from build123d import *

# Parameters (mm, degrees)
SKETCH1_R           = 2.75
BOSS_EXTRUDE1_DEPTH = 6.35
FILLET1_R           = 6.35
CHAMFER1_SIZE       = 3.175
SKETCH2_W           = 234.95
SKETCH2_H           = 12.7
BOSS_EXTRUDE2_DEPTH = 6.35


with BuildPart() as part:
    # Sketch1 → Boss-Extrude1 (new body)
    with BuildSketch(Plane.XY):
        with BuildLine():
            ThreePointArc((-19.05, 19.05), (-31.75, 6.35), (-19.05, -6.35))
            Line((-19.05, -6.35), (-19.05, -260.35))
            ThreePointArc((-19.05, -260.35), (-31.75, -273.05), (-19.05, -285.75))
            Line((-19.05, -285.75), (241.3, -285.75))
            ThreePointArc((241.3, -285.75), (254, -273.05), (241.3, -260.35))
            Line((241.3, -260.35), (241.3, -6.35))
            ThreePointArc((241.3, -6.35), (254, 6.35), (241.3, 19.05))
            Line((241.3, 19.05), (-19.05, 19.05))
        make_face()
        with Locations((241.3, 6.35)):
            Circle(SKETCH1_R, mode=Mode.SUBTRACT)
        with Locations((-19.05, -273.05)):
            Circle(SKETCH1_R, mode=Mode.SUBTRACT)
        with Locations((-9.525, -276.225)):
            Circle(SKETCH1_R, mode=Mode.SUBTRACT)
        with Locations((231.775, -276.225)):
            Circle(SKETCH1_R, mode=Mode.SUBTRACT)
        with Locations((241.3, -273.05)):
            Circle(SKETCH1_R, mode=Mode.SUBTRACT)
        with BuildLine():
            Line((-6.35, -247.65), (-6.35, -19.05))
            ThreePointArc((-6.35, -19.05), (6.35, -6.35), (-6.35, 6.35))
            Line((-6.35, 6.35), (228.6, 6.35))
            Line((228.6, 6.35), (228.6, -273.05))
            Line((228.6, -273.05), (-6.35, -273.05))
            ThreePointArc((-6.35, -273.05), (6.35, -260.35), (-6.35, -247.65))
        make_face(mode=Mode.SUBTRACT)
        with Locations((-6.35, -6.35)):
            Circle(SKETCH1_R, mode=Mode.SUBTRACT)
        with Locations((-6.35, -260.35)):
            Circle(SKETCH1_R, mode=Mode.SUBTRACT)
        with Locations((-19.05, 6.35)):
            Circle(SKETCH1_R, mode=Mode.SUBTRACT)
        with Locations((-9.525, 9.525)):
            Circle(SKETCH1_R, mode=Mode.SUBTRACT)
        with Locations((231.775, 9.525)):
            Circle(SKETCH1_R, mode=Mode.SUBTRACT)
    extrude(amount=BOSS_EXTRUDE1_DEPTH)

    # Fillet1
    fillet1_edges = [part.edges().sort_by_distance(p)[0] for p in [
        (228.6, -273.05, 3.175),
        (228.6, 6.35, 3.175),
        (-6.35, 6.35, 3.175),
    ]]
    fillet(fillet1_edges, radius=FILLET1_R)
    fillet1_2_edges = [part.edges().sort_by_distance(p)[0] for p in [
        (-6.35, -273.05, 3.175),
    ]]
    fillet(fillet1_2_edges, radius=FILLET1_R)

    # Chamfer1
    chamfer1_edges = [part.edges().sort_by_distance(p)[0] for p in [
        (-21.8, 6.35, 0),
        (-21.8, -273.05, 0),
        (238.55, 6.35, 0),
        (238.55, -273.05, 0),
        (-9.1, -260.35, 0),
        (-9.1, -6.35, 0),
    ]]
    chamfer(chamfer1_edges, length=CHAMFER1_SIZE)

    # Sketch2 → Boss-Extrude2 (add)
    with BuildSketch(Plane.XY.offset(6.35)):
        with Locations((111.125, -133.35)):
            Rectangle(SKETCH2_W, SKETCH2_H)
    extrude(amount=-BOSS_EXTRUDE2_DEPTH)


solid = part.part
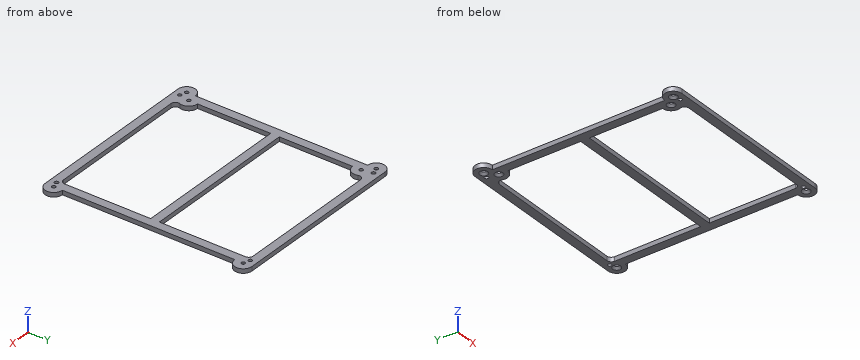
The listing builds one solid part. Answer for the finished solid, in the listing's coordinates (mm). Give positions to 0.01 mm unless a question says otherwise; leave off trailing zeros. Write each loop counter-clockwise with the first axis right and the second up, starting at its lowest first coordinate (ties: lowest second). Pieces come first, ordered by that corner, then holes. Notation, with made-up numbers: (52.25, 85) -> (90.25, 85) arc R20 cw to (90.25, 109) -> close; hole circle Ø10 at (6.5, 70.5). An arc over 180 degrees is marked (long way). One line per question, with ' | ' between items. Start each with the question number.
1. Find the intervals of material crossed by probe 1 along Y at (x, z) = (24, 0.75); probe 2 along X at (y, z) = (-126, 2.75), in increasing order.
2. Given pin 1 Ø7 at (x, y) = (241.3, 6.35) entering from -Z (3 decimals); pin 2 Ø3 at (y, z) = (-215.5, 4.5) entering from +X, each flat-ended and moving along its own axis, determine where each tip first touches the part or whether it passes through.
3. Section A-A (x = 210) is taken. Determine the outline of the cut face in (y, z).
4. Section B-B (y = -60.5) is taken. Determine the outline of the cut face in (x, z).
5. Section C-C (z = 4.75) is taken. State how many separate pieces and enclosed holes the cut face has, plus the area to 3 significant figures.
Response values:
1) probe 1: -285.75 to -273.05, -139.7 to -127, 6.35 to 19.05 | probe 2: -19.05 to -6.35, 228.6 to 241.3
2) pin 1: z = 2.425 | pin 2: x = 241.3
3) outline: (-285.75, 0) -> (-273.05, 0) -> (-273.05, 6.35) -> (-285.75, 6.35) -> close; (-139.7, 0) -> (-127, 0) -> (-127, 6.35) -> (-139.7, 6.35) -> close; (6.35, 0) -> (19.05, 0) -> (19.05, 6.35) -> (6.35, 6.35) -> close
4) outline: (-19.05, 0) -> (-6.35, 0) -> (-6.35, 6.35) -> (-19.05, 6.35) -> close; (228.6, 0) -> (241.3, 0) -> (241.3, 6.35) -> (228.6, 6.35) -> close
5) separate pieces: 1 | enclosed holes: 12 | area: 18,100 mm2
